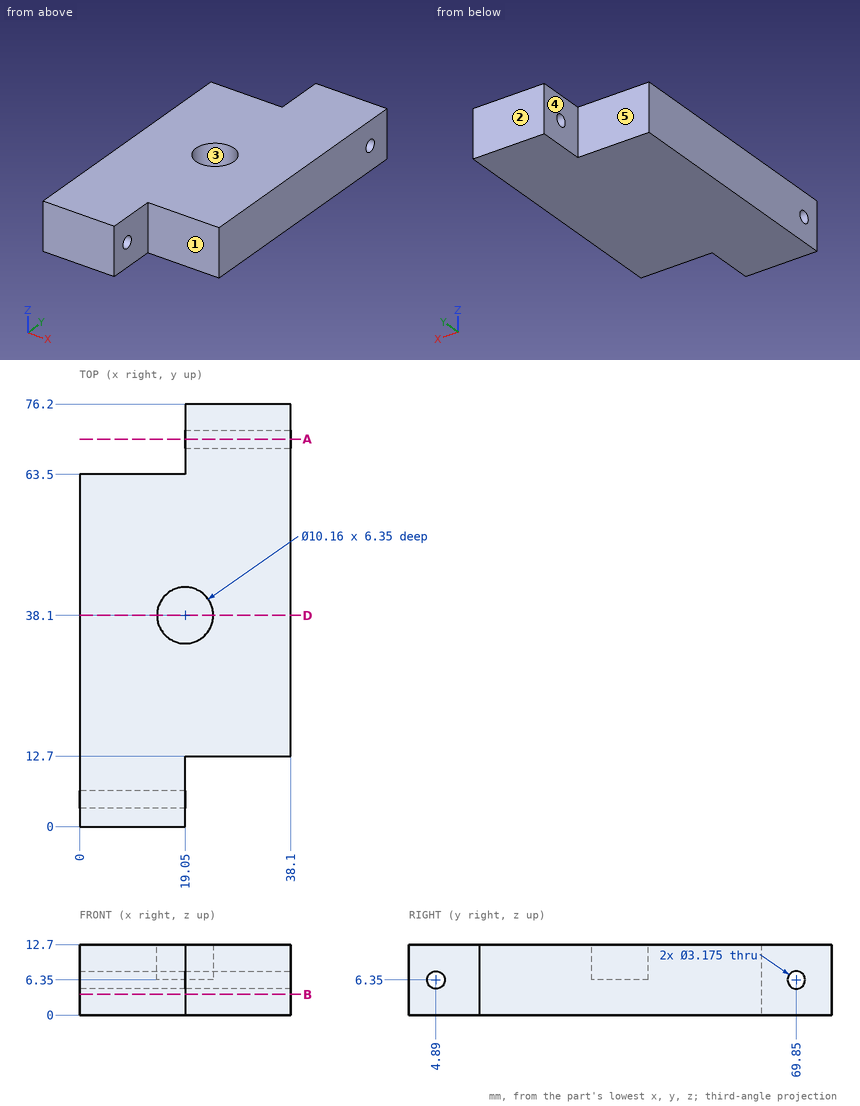
Verification items for this drawing (mm, ordinates from the low corner). A direction names the side the tool comes from. Coordinates: 2 decimals unless noted, no trailing zeros. Loops run counter-clockwise (first coordinate to the right, second up) from the corner with the lowest first, then second, coordinate; pieces in that order, holes last.
Item 1: Thickness scan on line 1 (Y direction, x = 16, z = 6.5); line 2 (Y direction, x = 24.25, z = 6.35); line 3 (Y direction, x = 13.5, z = 1.75). Record the ranges inside material, lowest first.
Item 2: Access from +Z, -Z, +X, -X, +Y, -Y to the whole of each face (thin tool, end or side, straight path). Record for the marked faces 1 and 2.
Item 3: Sectioned sample at B-B, the plane z = 3.75. Record the boundary of the cut face in (x, y), then the cut area to 3 significant figures.
Item 4: Go/stop test with flat-tipped pins: pin 1 Ø1 at (y, z) = (9.5, 9.5) entering from -X; pin 2 Ø4 at (x, z) = (10, 7) entering from +Y; pin 3 Ø6.5 at (y, z) = (67, 5) entering from -X; pin 4 Ø6.5 at (x, z) = (32.5, 8.5) entering from -Y. Record where each tip stops, or that it passes through.
Item 5: Release check for a two-part mould opening along Y. For the marked faces 3, 4 and 5 record: released by +Y, released by -Y, zero draft, split by the parting line, or undercut.
Item 6: Sectioned sample at D-D, the plane y = 38.1. Record the boundary of the cut face in (x, z).
Item 7: Sectioned sample at A-A, the plane y = 69.85. Record the boundary of the cut face in (x, z).
Check result:
1. line 1: y = 0 to 3.31, 6.47 to 34.04, 42.16 to 63.5
1. line 2: y = 12.7 to 68.26, 71.44 to 76.2
1. line 3: y = 0 to 63.5
2. face 1: +Z, -Z, +X, -Y
2. face 2: +Z, -Z, +X, -X, +Y
3. outline: (0, 0) - (19.05, 0) - (19.05, 12.7) - (38.1, 12.7) - (38.1, 76.2) - (19.05, 76.2) - (19.05, 63.5) - (0, 63.5) - close
3. area: 2,420 mm2
4. pin 1: stops at x = 0
4. pin 2: stops at y = 63.5
4. pin 3: stops at x = 19.05
4. pin 4: stops at y = 12.7
5. face 3: undercut
5. face 4: zero draft
5. face 5: released by +Y
6. outline: (0, 0) - (38.1, 0) - (38.1, 12.7) - (24.13, 12.7) - (24.13, 6.35) - (13.97, 6.35) - (13.97, 12.7) - (0, 12.7) - close
7. outline: (19.05, 0) - (38.1, 0) - (38.1, 4.76) - (19.05, 4.76) - close; (19.05, 7.94) - (38.1, 7.94) - (38.1, 12.7) - (19.05, 12.7) - close
